Input: part model. Units: mm. Frame: model coordinates. Coordinates: 2 decimals unless noted, no trailing zeros. Loops run counter-clockwise (first coordinate to the right, second up) from the corner with the lowest first, then second, coordinate; pieces in that order, holes last.
Autodesk Inventor part; units mm, degrees
ref_plane "YZ Plane" through (0, 0, 0) normal (1, 0, 0) x (0, 1, 0)
ref_plane "XZ Plane" through (0, 0, 0) normal (0, 1, 0) x (-1, 0, 0)
ref_plane "XY Plane" through (0, 0, 0) normal (0, 0, 1) x (1, 0, 0)
sketch "Sketch1" plane through (0, 0, 0) normal (0, 0, 1) x (1, 0, 0)
  line L0 (-200, 0) -> (-200, 150)
  line L1 (-200, 150) -> (200, 150)
  line L2 (200, 150) -> (200, 0)
  line L3 (200, 0) -> (-200, 0)
  line L4 (50, 150) -> (-50, 150)
  line L5 (-50, 150) -> (-50, 850)
  line L6 (-50, 850) -> (50, 850)
  line L7 (50, 850) -> (50, 150)
  line L8 (0, -170) -> (0, 1020)
  line L9 (-280, 0) -> (280, 0)
  point P0 (0, 0)
  dimension "d7" = 700
  dimension "d11" = 50
  dimension "d12" = 50
  dimension "d13" = 200
  dimension "d14" = 200
  dimension "d15" = 150
  dimension "d17" = 200
  dimension "d18" = 200
extrude "Extrusion2" add sketch "Sketch1" along normal blind 10
sketch "Sketch2" plane through (0, 0, 10) normal (0, 0, 1) x (1, 0, 0)
  line L0 (5, 140) -> (5, 740)
  line L1 (0, -170) -> (0, 1020)
  line L2 (-280, 0) -> (280, 0)
  arc A0 (0, 135) -> (5, 140) centre (0, 140) ccw
  line L3 (-5, 140) -> (-5, 740)
  arc A1 (-5, 140) -> (0, 135) centre (0, 140) ccw
  arc A2 (5, 740) -> (-5, 740) centre (0, 740) ccw
  line L4 (50, 850) -> (-50, 850)
  point P0 (0, 0)
  point P1 (0, 149.3301)
  dimension "d8" = 5
  dimension "d24" = 600
  dimension "d26" = 10
  dimension "d30" = 10
  dimension "d34" = 110
sketch "Sketch3" plane through (0, 0, 0) normal (0, 0, -1) x (-1, 0, 0)
  line L0 (0, -170) -> (0, 1020)
  line L1 (280, 0) -> (-280, 0)
  circle A0 centre (0, 810) radius 5
  line L2 (-50, 850) -> (50, 850)
  point P0 (0, 0)
  dimension "d19" = 10
  dimension "d27" = 40
extrude "Extrusion4" cut sketch "Sketch3" against normal through all
extrude "Extrusion6" cut sketch "Sketch2" against normal through all
Item 1: Section query C-C (x = 91). Output: boundary loops of the cut face in (y, z), then the cut area to 3 significant figures.
Result:
outline: (0, 0) - (150, 0) - (150, 10) - (0, 10) - close
area: 1,500 mm2
Item 2: Line query: L1, parallel to Y at x = 0, z = 2.75; L2, parallel to X at y = 440.5, z = 2.75; L3, parallel to X at y = 755, z = 1.5. Output: solid intervals per line, ascending.
Result:
L1: y = 0 to 135, 745 to 805, 815 to 850
L2: x = -50 to -5, 5 to 50
L3: x = -50 to 50
Item 3: Section query B-B (z = 6.75). Output: boundary loops of the cut face in (x, y), then the cut area to 3 significant figures.
Result:
outline: (-200, 0) - (200, 0) - (200, 150) - (50, 150) - (50, 850) - (-50, 850) - (-50, 150) - (-200, 150) - close; hole (-5, 140) arc R5 ccw to (5, 140) - (5, 740) arc R5 ccw to (-5, 740) - close; hole circle Ø10 at (0, 810)
area: 124,000 mm2
Item 4: Section query A-A (y = 314.5). Output: boundary loops of the cut face in (x, z), then the cut area to 3 significant figures.
Result:
outline: (-50, 0) - (-5, 0) - (-5, 10) - (-50, 10) - close; (5, 0) - (50, 0) - (50, 10) - (5, 10) - close
area: 900 mm2
Item 5: Contact query for flat-ended pins moving along their axis: P1, Ø5, axis at y = 390.5, z = 7.5, coming from the +X side; P2, Ø1, axis at x = -99.5, z = 1, coming from the +Y side; P3, Ø5, axis at y = 463, z = 4.5, coming from the -X side. Output: stop coordinate, or through.
Result:
P1: stops at x = 50
P2: stops at y = 150
P3: stops at x = -50
